Check sheet for the modelled part. Datum: model origin and axes. Units: mm. A direction names the side the tool comes from. Round coordinates to 2 decimals unless told otherwise and drop trailing zeros. Write each loop counter-clockwise with the first axis right and the second up, starting at its lowest first coordinate (ties: lowest second). Pieces come first, ordered by that corner, then holes. Notation, with made-up numbers: M 89.25,-9.5 L 140.25,-9.5 A19 ccw 140.25,8.5 Z; hole C 60.25,80.5 d7. An arc over 180 degrees is marked long. Answer in a Markdown table with one row per item.
Autodesk Fusion 360 part; units mm, degrees
sketch "Sketch1" plane through (0, 0, 0) normal (0, 1, 0) x (1, 0, 0)
  line L0 (25, -12.5) -> (-25, -12.5)
  line L1 (-25, -12.5) -> (-25, 12.5)
  line L2 (-25, 12.5) -> (25, 12.5)
  line L3 (25, 12.5) -> (25, -12.5)
  line L4 (25, -12.5) -> (-25, 12.5) construction
  line L5 (-25, -12.5) -> (25, 12.5) construction
  dimension "d1" = 25
  dimension "d2" = 50
extrude "Extrude1" add sketch "Sketch1" along normal blind 35
sketch "Sketch2" plane through (0, 0, 12.5) normal (0, 0, 1) x (1, 0, 0)
  line L0 (-25, 0) -> (25, 0)
  line L1 (25, 0) -> (25, 35)
  line L2 (25, 35) -> (-25, 35)
  line L3 (-25, 35) -> (-25, 0)
  line L4 (0, 0) -> (0, 11) construction
  line L5 (23, 35) -> (22.15, 34.1)
  line L6 (22.15, 34.1) -> (22.15, 33.5)
  line L7 (22.15, 33.5) -> (23.15, 33.5)
  line L8 (23.15, 33.5) -> (23.15, 29)
  line L9 (23.15, 29) -> (0, 29)
  line L10 (23, 35) -> (0, 35)
  line L11 (-25, 35) -> (25, 35)
  line L12 (-23.15, 33.5) -> (-23.15, 29)
  line L13 (-25, 0) -> (-25, 35)
  line L14 (-23, 35) -> (0, 35)
  line L15 (-22.15, 33.5) -> (-23.15, 33.5)
  line L16 (-22.15, 34.1) -> (-22.15, 33.5)
  line L17 (-23.15, 29) -> (0, 29)
  line L18 (-23, 35) -> (-22.15, 34.1)
  dimension "d5" = 46.3
  dimension "d6" = 1
  dimension "d7" = 1.5
  dimension "d8" = 0.6
  dimension "d9" = 2
  dimension "d10" = 4.5
extrude "Extrude2" cut sketch "Sketch2" against normal through all contours L2 L5 L6 L7 L8 L9 L10 L11 L12 L14 L15 L16 L17 L18
sketch "Sketch3" plane through (0, 0, 12.5) normal (0, 0, 1) x (1, 0, 0)
  line L0 (23, 35) -> (22.15, 34.1)
  line L1 (22.15, 34.1) -> (22.15, 33.5)
  line L2 (22.15, 33.5) -> (23.15, 33.5)
  line L3 (23.15, 33.5) -> (23.15, 29)
  line L4 (23.15, 29) -> (-23.15, 29)
  line L5 (-23.15, 29) -> (-23.15, 33.5)
  line L6 (-23.15, 33.5) -> (-22.15, 33.5)
  line L7 (-22.15, 33.5) -> (-22.15, 34.1)
  line L8 (-22.15, 34.1) -> (-23, 35)
  line L9 (-23, 35) -> (-25, 35)
  line L10 (-25, 35) -> (-25, 0)
  line L11 (-25, 0) -> (25, 0)
  line L12 (25, 0) -> (25, 35)
  line L13 (25, 35) -> (23, 35)
  line L14 (6, 23.5) -> (-6, 23.5)
  line L15 (-6, 23.5) -> (-6, 34.5)
  line L16 (-6, 34.5) -> (6, 34.5)
  line L17 (6, 34.5) -> (6, 23.5)
  line L18 (6, 23.5) -> (-6, 34.5) construction
  line L19 (-6, 23.5) -> (6, 34.5) construction
  point P0 (0, 29)
  dimension "d12" = 12
  dimension "d13" = 11
extrude "Extrude3" cut sketch "Sketch3" against normal blind 5 contours L4 L14 L15 L17
sketch "Sketch4" plane through (25, 0, 0) normal (1, 0, 0) x (0, 0, -1)
  line L0 (-12.5, 0) -> (12.5, 0)
  line L1 (12.5, 0) -> (12.5, 35)
  line L2 (12.5, 35) -> (-12.5, 35)
  line L3 (-12.5, 35) -> (-12.5, 0)
  line L4 (-12.5, 17.5) -> (12.5, 0)
  line L5 (12.5, 0) -> (-12.5, 0)
  line L6 (-12.5, 0) -> (-12.5, 17.5)
extrude "Extrude4" cut sketch "Sketch4" against normal through all contours L0 L3 L4 L5 L6
sketch "Sketch5" plane through (0, 0, 12.5) normal (0, 0, 1) x (1, 0, 0)
  line L0 (-25, 17.5) -> (25, 17.5)
  line L1 (25, 17.5) -> (25, 35)
  line L2 (25, 35) -> (23, 35)
  line L3 (23, 35) -> (22.15, 34.1)
  line L4 (22.15, 34.1) -> (22.15, 33.5)
  line L5 (22.15, 33.5) -> (23.15, 33.5)
  line L6 (23.15, 33.5) -> (23.15, 29)
  line L7 (23.15, 29) -> (6, 29)
  line L8 (6, 29) -> (6, 23.5)
  line L9 (6, 23.5) -> (-6, 23.5)
  line L10 (-6, 23.5) -> (-6, 29)
  line L11 (-6, 29) -> (-23.15, 29)
  line L12 (-23.15, 29) -> (-23.15, 33.5)
  line L13 (-23.15, 33.5) -> (-22.15, 33.5)
  line L14 (-22.15, 33.5) -> (-22.15, 34.1)
  line L15 (-22.15, 34.1) -> (-23, 35)
  line L16 (-23, 35) -> (-25, 35)
  line L17 (-25, 35) -> (-25, 17.5)
  line L18 (23, 19.5) -> (-23, 19.5)
  line L19 (-23, 19.5) -> (-23, 0)
  line L20 (-23, 0) -> (23, 0)
  line L21 (23, 0) -> (23, 19.5)
  line L22 (23, 19.5) -> (-23, 0) construction
  line L23 (-23, 19.5) -> (23, 0) construction
  line L24 (-25, 0) -> (25, 0)
  line L25 (25, 17.5) -> (25, 0)
  line L26 (-25, 0) -> (-25, 17.5)
  point P0 (0, 9.75)
  dimension "d17" = 2
  dimension "d18" = 2
  dimension "d19" = 2
extrude "Extrude5" cut sketch "Sketch5" against normal blind 21 contours L0 L18 L19 L21 | L0 L19 L20 L21 L24
sketch "Sketch6" plane through (0, 0, -8.5) normal (0, 0, 1) x (1, 0, 0)
  line L0 (-23, 2.8) -> (23, 2.8)
  line L1 (23, 2.8) -> (23, 19.5)
  line L2 (23, 19.5) -> (-23, 19.5)
  line L3 (-23, 19.5) -> (-23, 2.8)
  circle A0 centre (0, 9.5) radius 3.25
  line L4 (0, 0) -> (0, 14) construction
  dimension "d22" = 6.5
  dimension "d23" = 9.5
extrude "Extrude6" cut sketch "Sketch6" against normal through all contours A0
1. Draft check along X on faces 6 (the face through (-0.423, 12.722, -10.472)), 7 (the face through (-25, 21, 0)), 8 (the face through (24, 35, 0)). Enter one of: +X half, -X half, draft (parallel to the pull), parting line (faces both ways), or undercut.
Found:
| item | result |
|---|---|
| face 6 | undercut |
| face 7 | -X half |
| face 8 | draft |
2. Section check C-C, the plane y = 18.5. Record the cut outline in (x, z), and give its area (3 significant figures).
Found:
| item | result |
|---|---|
| outline | M -25,-12.5 L 25,-12.5 L 25,12.5 L 23,12.5 L 23,-8.5 L -23,-8.5 L -23,12.5 L -25,12.5 Z |
| area | 284 mm2 |
3. Section check A-A, the plane x = 0. Record the cut outline in (y, z), and give its area (3 significant figures).
Found:
| item | result |
|---|---|
| outline | M 0,-12.5 L 6.25,-12.5 L 6.25,-8.5 L 2.8,-8.5 Z; M 12.75,-12.5 L 29,-12.5 L 29,7.5 L 23.5,7.5 L 23.5,12.5 L 19.5,12.5 L 19.5,-8.5 L 12.75,-8.5 Z |
| area | 256 mm2 |
4. Section check B-B, the plane y = 12. Record the cut outline in (x, z).
Found:
| item | result |
|---|---|
| outline | M -25,-12.5 L -2.08,-12.5 L -2.08,-8.5 L -23,-8.5 L -23,4.64 L -25,4.64 Z; M 2.08,-12.5 L 25,-12.5 L 25,4.64 L 23,4.64 L 23,-8.5 L 2.08,-8.5 Z |
5. Section check D-D, the plane z = -5. Record the cut outline in (x, y), and give its area (3 significant figures).
Found:
| item | result |
|---|---|
| outline | M -25,5.25 L -23,5.25 L -23,19.5 L 23,19.5 L 23,5.25 L 25,5.25 L 25,35 L 23,35 L 22.15,34.1 L 22.15,33.5 L 23.15,33.5 L 23.15,29 L -23.15,29 L -23.15,33.5 L -22.15,33.5 L -22.15,34.1 L -23,35 L -25,35 Z |
| area | 556 mm2 |
6. Go/stop test with flat-tipped pins: pin 1 (2 mm diameter, centred on x = 12.5, z = -2, fed in from +Y); pin 2 (6.5 mm diameter, centred on x = 9.5, z = 5, fed in from -Y); pin 3 (0.5 mm diameter, centred on x = -23, z = -2.5, fed in from -Y) (3 decimals). Record where each tip stops, or that it passes through.
Found:
| item | result |
|---|---|
| pin 1 | stops at y = 29 |
| pin 2 | stops at y = 19.5 |
| pin 3 | stops at y = 6.825 |
7. Scan lines: L1, parallel to X at y = 27, z = 10.5; L2, parallel to Z at x = -9.5, y = 9.5; L3, parallel to Y at x = -20.5, z = 3.75. Record each from-to range of solid material in increasing order.
Found:
| item | result |
|---|---|
| L1 | x = -25 to -6, 6 to 25 |
| L2 | z = -12.5 to -8.5 |
| L3 | y = 19.5 to 29 |
8. Access from +Z, -Z, +X, -X, +Y, -Y to the whole of each face (thin tool, end or side, straight path). Record for faces 1 (the face through (25, 21, 0)), 2 (the face through (0, 23.5, 10)), 3 (the face through (0, 22, 12.5)), 4 (the face through (23.15, 31, 0)), 5 (the face through (-23, 13, 0)).
Found:
| item | result |
|---|---|
| face 1 | +Z, -Z, +X, +Y, -Y |
| face 2 | +Z, +Y |
| face 3 | +Z, +X, -X, +Y, -Y |
| face 4 | +Z, -Z |
| face 5 | +Z, -Y |
